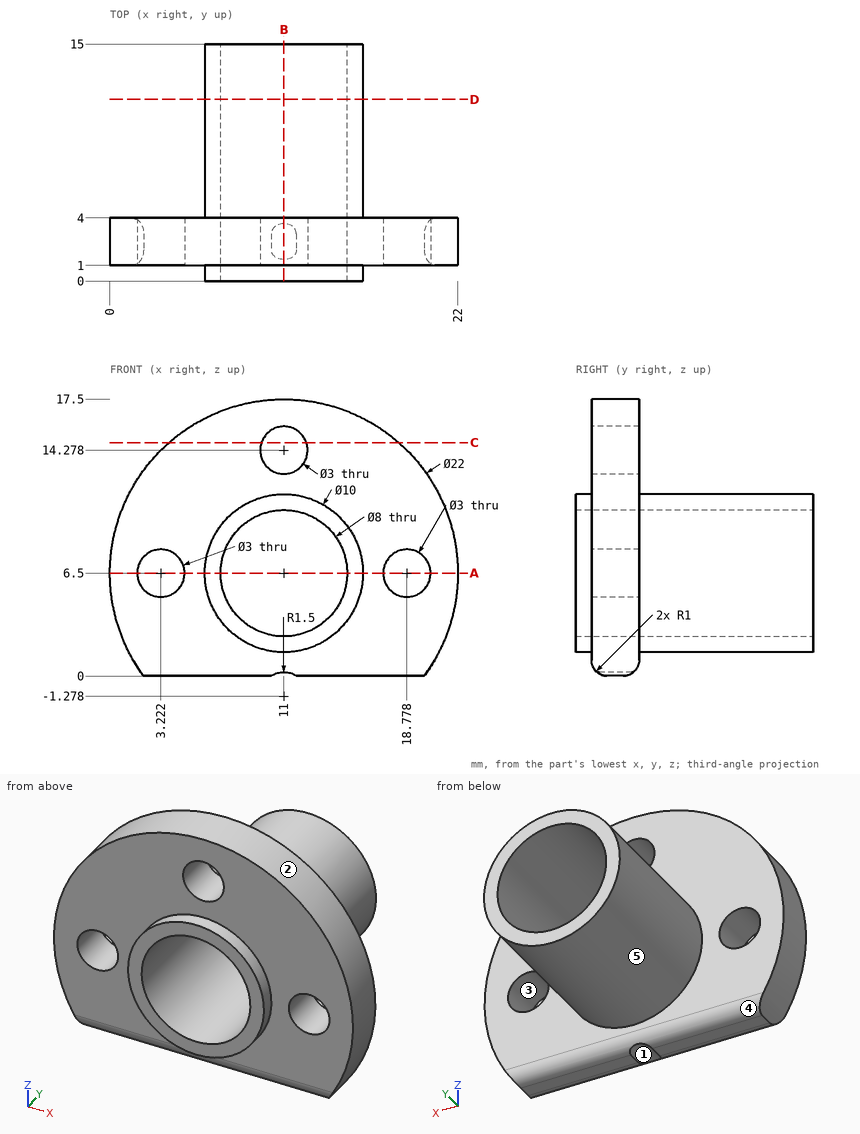
Source: three-view drawing plus pictorial views. Frame: mm from the lowest corner of the part. A direction names the side the tool comes from. Round coordinates to 2 decimals unless told otherwise and drop trailing zeros. Loops run counter-clockwise (first coordinate to the right, second up) from the corner with the lowest first, then second, coordinate; pieces in that order, holes last. Notation, with made-up numbers: (-7, 88.5) - (16, 88.5) arc R13 ccw to (16, 102.5) - close; hole circle Ø8 at (-8.75, 66.25). An arc over 180 degrees is marked (long way). Write item = value, one per line. Start each with the question number.
Item 1: Reachability of the marked faces 4 and 5 from +Z, -Z, +X, -X, +Y, -Y: full face, straight path, thin tool, end or side. Return the list, or none.
Item 2: Section query C-C on z = 14.75. Output: boundary loops of the cut face in (x, y), plus the area to 3 significant figures.
Item 3: Section query B-B on x = 11. Output: boundary loops of the cut face in (y, z).
Item 4: First-contact query: pin 1 Ø2 at (x, z) = (16, 10.5) entering from +Y; pin 2 Ø3 at (y, z) = (9, 2.5) entering from +X; pin 3 Ø8 at (y, z) = (8.5, 9) entering from +X; pin 4 Ø7 at (x, z) = (11, 6.5) entering from -Y. Flat tips, straight axial feed; report the tip coordinate or a pass-through.
Item 5: Material intervals for line 1 (X direction, y = 3.05, z = 6.5); line 2 (X direction, y = 9.5, z = 6.5); line 3 (X direction, y = 3.25, z = 13) (1 decimal), sorted ascending.
Item 6: Mould query, pull axis Z, two halves, no side actions, for the marked faces 1, 2 and 3. Classes: released by +Z, released by -Z, zero draft, split by the parting line, or undercut.
Item 7: Section query D-D on y = 11.5. Output: boundary loops of the cut face in (x, z), plus the area to 3 significant figures.
Item 8: Section query A-A on z = 6.5. Output: boundary loops of the cut face in (x, y).
Results list:
q1.face_4 = -Z, +X, -X, +Y
q1.face_5 = +Y
q2.outline = (3.72, 1) - (9.58, 1) - (9.58, 4) - (3.72, 4) - close; (12.42, 1) - (18.28, 1) - (18.28, 4) - (12.42, 4) - close
q2.area = 35.1 mm²
q3.outline = (0, 1.5) - (1, 1.5) - (1, 1) arc R1 ccw to (1.37, 0.22) - (3.63, 0.22) arc R1 ccw to (4, 1) - (4, 1.5) - (15, 1.5) - (15, 2.5) - (0, 2.5) - close; (0, 10.5) - (15, 10.5) - (15, 11.5) - (4, 11.5) - (4, 12.78) - (1, 12.78) - (1, 11.5) - (0, 11.5) - close; (1, 15.78) - (4, 15.78) - (4, 17.5) - (1, 17.5) - close
q4.pin_1 = 4
q4.pin_2 = 15.33
q4.pin_3 = 16
q4.pin_4 = through
q5.line_1 = 0 to 1.72, 4.72 to 7, 15 to 17.28, 20.28 to 22
q5.line_2 = 6 to 7, 15 to 16
q5.line_3 = 2.1 to 10.2, 11.8 to 19.9
q6.face_1 = released by -Z
q6.face_2 = split by the parting line
q6.face_3 = undercut
q7.outline = circle Ø10 at (11, 6.5); hole circle Ø8 at (11, 6.5)
q7.area = 28.3 mm²
q8.outline = (0, 1) - (1.72, 1) - (1.72, 4) - (0, 4) - close; (4.72, 1) - (6, 1) - (6, 0) - (7, 0) - (7, 15) - (6, 15) - (6, 4) - (4.72, 4) - close; (15, 0) - (16, 0) - (16, 1) - (17.28, 1) - (17.28, 4) - (16, 4) - (16, 15) - (15, 15) - close; (20.28, 1) - (22, 1) - (22, 4) - (20.28, 4) - close
